Read the model definition and answer for the solid it produces. Units are mm, in the model's axes. A direction names the side the tool comes from. Round coordinates to 2 decimals unless told otherwise and drop trailing zeros. Loops run counter-clockwise (first coordinate to the right, second up) from the corner with the lowest first, then second, coordinate; pieces in that order, holes last. Notation, with made-up numbers: (-20, 79) - (-3, 79) arc R20 cw to (-3, 118) - close; hole circle Ø6 at (-34, 86.25). An arc over 180 degrees is marked (long way). Answer as CSV lines item,"result".
```python
from build123d import *

# Parameters (mm, degrees)
CROQUIS1_R              = 3.5
SALIENTE_EXTRUIR1_DEPTH = 52.5
SALIENTE_EXTRUIR2_START = -3
CROQUIS2_R              = 29.5
CROQUIS2_R_2            = 1.75
SALIENTE_EXTRUIR2_DEPTH = 3
CORTAR_EXTRUIR1_DEPTH   = 79.744841101
CORTAR_EXTRUIR2_DEPTH   = 79.744841101
CORTAR_EXTRUIR3_DEPTH   = 79.744841101
CROQUIS7_W              = 12.05
CROQUIS7_H              = 3.5
CORTAR_EXTRUIR4_DEPTH   = 79.744841101
CROQUIS8_W              = 98.89383178
CROQUIS8_H              = 87.653821396
CORTAR_EXTRUIR5_DEPTH   = 49.5


with BuildPart() as part:
    # Croquis1 → Saliente-Extruir1 (new body)
    with BuildSketch(Plane.XY):
        with BuildLine():
            Line((-39.727194716, -12), (-26.949025956, -12))
            ThreePointArc((-26.949025956, -12), (0, 29.5), (26.949025956, -12))
            Line((26.949025956, -12), (39.727194716, -12))
            ThreePointArc((39.727194716, -12), (0, 41.5), (-39.727194716, -12))
        make_face()
        with Locations((-35.5, 0)):
            Circle(CROQUIS1_R, mode=Mode.SUBTRACT)
        with Locations((0, 35.5)):
            Circle(CROQUIS1_R, mode=Mode.SUBTRACT)
        with Locations((35.5, 0)):
            Circle(CROQUIS1_R, mode=Mode.SUBTRACT)
    extrude(amount=SALIENTE_EXTRUIR1_DEPTH)

    # Croquis2 → Saliente-Extruir2 (add)
    with BuildSketch(Plane.XY.offset(52.5).offset(SALIENTE_EXTRUIR2_START)):
        Circle(CROQUIS2_R)
        with Locations((-8.025, 8.025)):
            Circle(CROQUIS2_R_2, mode=Mode.SUBTRACT)
        with Locations((8.025, 8.025)):
            Circle(CROQUIS2_R_2, mode=Mode.SUBTRACT)
        with Locations((-8.025, -8.025)):
            Circle(CROQUIS2_R_2, mode=Mode.SUBTRACT)
        with Locations((8.025, -8.025)):
            Circle(CROQUIS2_R_2, mode=Mode.SUBTRACT)
    extrude(amount=SALIENTE_EXTRUIR2_DEPTH)

    # Croquis3 → Cortar-Extruir1 (cut, through all)
    with BuildSketch(Plane.XY.offset(52.5)):
        with BuildLine():
            Line((-8.025, 6.025), (-8.025, -6.025))
            ThreePointArc((-8.025, -6.025), (-6.610786438, -6.610786438), (-6.025, -8.025))
            Line((-6.025, -8.025), (6.025, -8.025))
            ThreePointArc((6.025, -8.025), (6.610786438, -6.610786438), (8.025, -6.025))
            Line((8.025, -6.025), (8.025, 6.025))
            ThreePointArc((8.025, 6.025), (6.610786438, 6.610786438), (6.025, 8.025))
            Line((6.025, 8.025), (-6.025, 8.025))
            ThreePointArc((-6.025, 8.025), (-6.610786438, 6.610786438), (-8.025, 6.025))
        make_face()
    extrude(amount=-CORTAR_EXTRUIR1_DEPTH, mode=Mode.SUBTRACT)

    # Croquis5 → Cortar-Extruir2 (cut, through all)
    with BuildSketch(Plane.XY.offset(52.5)):
        Polygon((-26.949025956, -12), (26.949025956, -12), (26.949025956, -33.158311757), (-29.290832667, -29.730661126), align=None)
    extrude(amount=-CORTAR_EXTRUIR2_DEPTH, mode=Mode.SUBTRACT)

    # Croquis6 → Cortar-Extruir3 (cut, through all)
    with BuildSketch(Plane.XY.offset(52.5)):
        with BuildLine():
            Line((-40.277164746, 10), (-13.698766072, 10))
            ThreePointArc((-13.698766072, 10), (-11.992835192, 11.992835192), (-10, 13.698766072))
            Line((-10, 13.698766072), (-10, 40.277164746))
            ThreePointArc((-10, 40.277164746), (-29.344931419, 29.344931419), (-40.277164746, 10))
        make_face()
        with BuildLine():
            Line((10, 13.698766072), (10, 40.277164746))
            ThreePointArc((10, 40.277164746), (29.344931419, 29.344931419), (40.277164746, 10))
            Line((40.277164746, 10), (13.698766072, 10))
            ThreePointArc((13.698766072, 10), (11.992835192, 11.992835192), (10, 13.698766072))
        make_face()
    extrude(amount=-CORTAR_EXTRUIR3_DEPTH, mode=Mode.SUBTRACT)

    # Croquis7 → Cortar-Extruir4 (cut, through all)
    with BuildSketch(Plane.XY.offset(52.5)):
        with Locations((0, 9.775)):
            Rectangle(CROQUIS7_W, CROQUIS7_H)
        with Locations((0, -9.775)):
            Rectangle(CROQUIS7_W, CROQUIS7_H)
    extrude(amount=-CORTAR_EXTRUIR4_DEPTH, mode=Mode.SUBTRACT)

    # Croquis8 → Cortar-Extruir5 (cut)
    with BuildSketch(Plane(origin=(0, 0, 0), x_dir=(-1, 0, 0), z_dir=(0, 0, -1))):
        Rectangle(CROQUIS8_W, CROQUIS8_H)
    extrude(amount=-CORTAR_EXTRUIR5_DEPTH, mode=Mode.SUBTRACT)


solid = part.part
```
1) A cutting plane is placed at C-C, the plane y = 0. Determine the outline of the cut face in (x, z) (3 decimals), plus the area to 3 significant figures.
Entries:
outline,"(-41.5, 49.5) - (-39, 49.5) - (-39, 52.5) - (-41.5, 52.5) - close; (-32, 49.5) - (-8.025, 49.5) - (-8.025, 52.5) - (-32, 52.5) - close; (8.025, 49.5) - (32, 49.5) - (32, 52.5) - (8.025, 52.5) - close; (39, 49.5) - (41.5, 49.5) - (41.5, 52.5) - (39, 52.5) - close"
area,"159 mm^2"
2) A cutting plane is placed at A-A, the plane x = -35.5. Determine the outline of the cut face in (y, z).
Entries:
outline,"(-12, 49.5) - (-3.5, 49.5) - (-3.5, 52.5) - (-12, 52.5) - close; (3.5, 49.5) - (10, 49.5) - (10, 52.5) - (3.5, 52.5) - close"
3) A tool of negligible diameter and unlimited length cuts with its end or side. For faces 4 (the face through (10, 27, 51)), 5 (the face through (8.025, 0, 51)), 6 (the face through (-27, 10, 51)), 7 (the face through (-1, 15, 52.5)), from which of +Z, -Z, +X, -X, +Y, -Y can it reach the whole face along a straight path? Write none if from no direction.
Entries:
face 4,"+Z, -Z, +X, +Y"
face 5,"+Z, -Z"
face 6,"+Z, -Z, -X, +Y"
face 7,"+Z, +X, -X, +Y, -Y"
4) A cutting plane is placed at D-D, the plane z = 50.2. Count the separate pieces of the cut face and the enclosed holes in it, plus the area to 3 significant figures.
Entries:
separate pieces,"1"
enclosed holes,"8"
area,"1,960 mm^2"
5) Each of these flat-tipped pins is pushed along its axis until it touches: P1, Ø0.9, axis at x = 2.5, z = 51, coming from the +Y side; P2, Ø1.5, axis at x = 28, z = 51, coming from the +Y side; P3, Ø0.9, axis at y = -10, z = 51, coming from the -X side. Where does it stop, or does it pass through?
Entries:
P1,"stops at y = 41.45"
P2,"stops at y = 10"
P3,"stops at x = -40.39"
6) The mould has two halves that part along Y. Classify faces 1 (the face through (-10, 27, 51)), 2 (the face through (32.7, -2.1, 51)), 3 (the face through (-1, -12, 51)): pulls with the +Y half, pulls with the -Y half, needs draft (parallel to the pull), parting line crosses it, or undercut.
Entries:
face 1,"needs draft"
face 2,"undercut"
face 3,"pulls with the -Y half"
7) Find the intervals of material crossed by line 1 (Y direction, x = 35.5, z = 51.05); line 2 (X direction, y = -10, z = 49.6) (3 decimals); line 3 (X direction, y = 0, z = 50.2) (3 decimals), in increasing order.
Entries:
line 1,"y = -12 to -3.5, 3.5 to 10"
line 2,"x = -40.277 to -6.025, 6.025 to 40.277"
line 3,"x = -41.5 to -39, -32 to -8.025, 8.025 to 32, 39 to 41.5"
8) A cutting plane is placed at B-B, the plane y = 35.5. Determine the outline of the cut face in (x, z), plus the area to 3 significant figures.
Entries:
outline,"(-10, 49.5) - (-3.5, 49.5) - (-3.5, 52.5) - (-10, 52.5) - close; (3.5, 49.5) - (10, 49.5) - (10, 52.5) - (3.5, 52.5) - close"
area,"39.0 mm^2"
